Autodesk Inventor part; units mm, degrees
ref_plane "Work Plane1" through (32.5, 157, 0) normal (1, 0, 0) x (0, 1, 0)
ref_plane "XZ Plane" through (0, 0, 0) normal (0, 1, 0) x (-1, 0, 0)
ref_plane "XY Plane" through (0, 0, 0) normal (0, 0, 1) x (1, 0, 0)
sketch "Sketch1" plane through (0, 0, 0) normal (0, 1, 0) x (-1, 0, 0)
  circle A0 centre (0, 0) radius 19
  dimension "d0" = 38
extrude "Extrusion1" add sketch "Sketch1" along normal blind 157
sketch "Sketch2" plane through (0, 157, 0) normal (0, 1, 0) x (1, 0, 0)
  circle A0 centre (0, 0) radius 32.5
  dimension "d3" = 65
extrude "Extrusion2" add sketch "Sketch2" along normal blind 70
sketch "Sketch3" plane through (0, 227, 0) normal (0, 1, 0) x (1, 0, 0)
  circle A0 centre (0, 0) radius 11
  dimension "d6" = 22
extrude "Extrusion3" add sketch "Sketch3" along normal blind 13
chamfer "Chamfer1" distance 10 angle 45 2 edges at (-32.5, 227, 0) (-32.5, 157, 0)
chamfer "Chamfer2" distance 2 angle 45 1 edges at (19, 0, 0)
thread "Thread1"
sketch "Sketch5" plane through (0, 240, 0) normal (0, 1, 0) x (1, 0, 0)
  point P0 (0, 0)
  point P1 (0, 0)
hole "Hole1" at (0, 240, 0) direction (0, -1, 0) diameter 10.106 depth 35 tip angle 118
ref_plane "Work Plane1" through (32.5, 157, 0) normal (1, 0, 0) x (0, 1, 0)
sketch "Sketch8" plane through (32.5, 157, 0) normal (1, 0, 0) x (0, 1, 0)
  line L0 (60, -32.5) -> (60, 32.5)
  line L1 (10, -32.5) -> (60, -32.5)
  line L2 (10, 32.5) -> (10, -32.5)
  line L3 (10, 32.5) -> (60, 32.5)
  line L4 (60, 32.5) -> (10, -32.5) construction
  line L5 (60, -32.5) -> (10, 32.5) construction
  point P0 (-157, 0)
  point P1 (35, 0)
hole "Hole3" at (32.5, 192, 0) direction (-1, 0, 0) diameter 12 end through all
properties part number "screw.spindle" material "Steel, High Strength, Low Alloy"
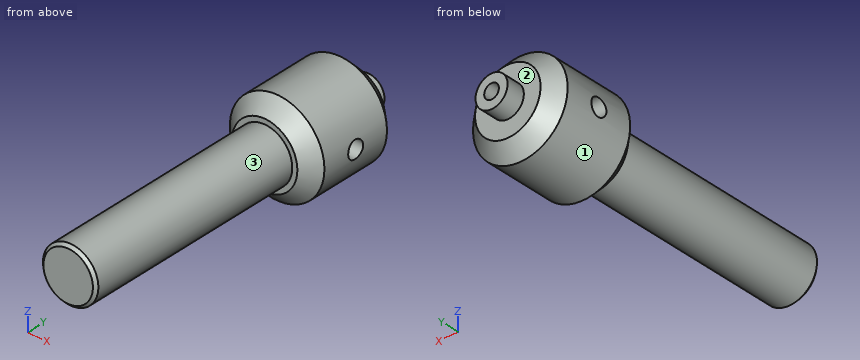
CAD build for the part. Positions are in the model's coordinates, mm. Face numbers are marked on the shaded views. A direction names the side the tool comes from. Round coordinates to 2 decimals unless told otherwise and drop trailing zeros. Order: outer loops, then holes, each group sorted by start corner. A loop starts at its lowest first (then second) coordinate and runs counter-clockwise, first axis right, second up. Notation, with made-up numbers: (33.5, 61) - (59.5, 61) arc R5 cw to (59.5, 68) - close; hole circle Ø9 at (14, 9.25). An arc over 180 degrees is marked (long way). Use CSV: the item, a comma, the result in double quotes. Start each with the question number.
1) Pin check, flat tips, straight feed: pin 1 Ø6 at (y, z) = (168.5, -17.5) entering from -X; pin 2 Ø11 at (y, z) = (192, 0) entering from +X; pin 3 Ø1 at (x, z) = (14, -6) entering from +Y; pin 4 Ø2 at (y, z) = (40.5, 16) entering from +X. Stop position of each tip, or through.
2) Tool access for the marked faces 1, 2 and 3: list every direction of +Z, -Z, +X, -X, +Y, -Y with a clear straight run to the whole face (end or side of a thin tool).
3) Saw through at B-B (y = 106.5). List the corners of the cut face in (x, z).
4) Wall check: L1, parallel to Z at x = 1, y = 192; L2, parallel to Y at x = 14, z = 0; L3, parallel to X at y = 228, z = 0. Give the ranges that are in metal, low to high. Write a range as [from, to].
5) Saw through at A-A (y = 192). List the corners of the cut face in (x, z).
Values follow:
1,pin 1,"stops at x = -29.09"
1,pin 2,"passes through"
1,pin 3,"stops at y = 227"
1,pin 4,"stops at x = 11.66"
2,face 1,"+Y, -Y"
2,face 2,"+Y"
2,face 3,"-Y"
3,outline,"circle Ø38 at (0, 0)"
4,L1,"z = [-32.48, -6], [6, 32.48]"
4,L2,"y = [0, 186], [198, 227]"
4,L3,"x = [-11, -5.05], [5.05, 11]"
5,outline,"(-31.94, -6) arc R32.5 ccw to (31.94, -6) - close; (-31.94, 6) - (31.94, 6) arc R32.5 ccw to start"
